Drawing for the job (mm, zero at the part's lowest x, y, z). A direction names the side the tool comes from. Round coordinates to 2 decimals unless told otherwise and drop trailing zeros. Loops run counter-clockwise (first coordinate to the right, second up) from the corner with the lowest first, then second, coordinate; pieces in that order, holes last. Notation, with made-up numbers: M -21.5,36 L 11.5,36 A15 ccw 11.5,64 Z; hole C 31.5,69.25 d4. An arc over 180 degrees is marked long. Put each result on its own line as item: value. Start each with the question number.
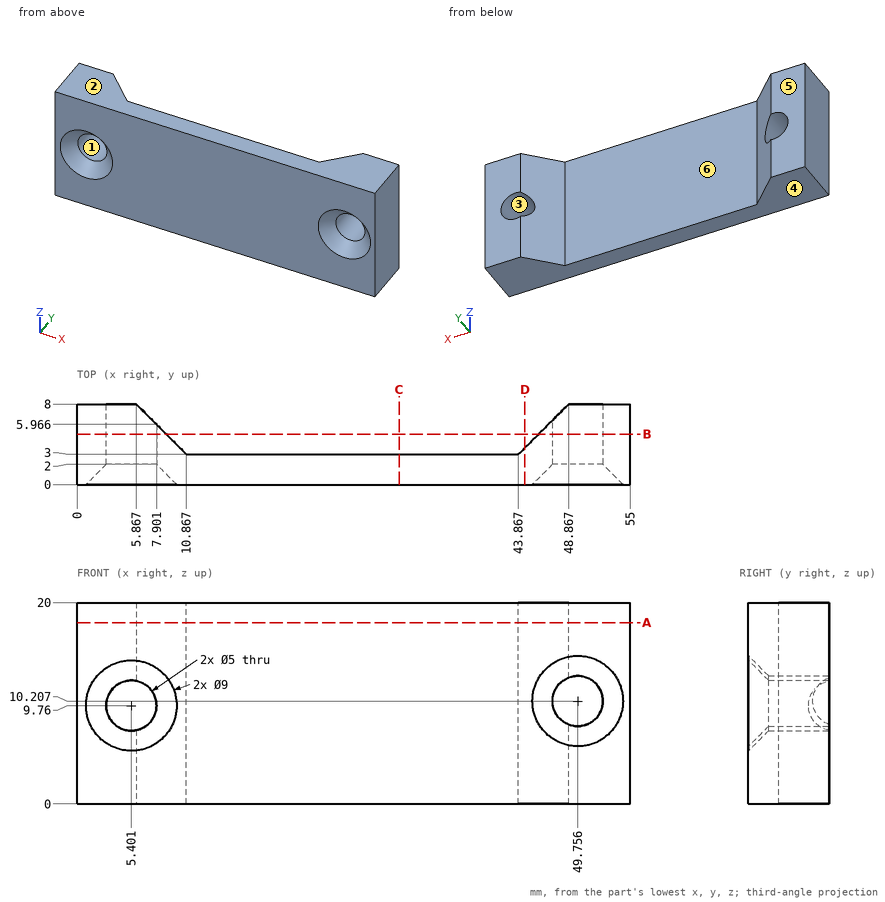
1. Cut at C-C, the plane x = 32. Give the cut face in (y, z).
2. Cut at B-B, the plane y = 5. Give the cut face in (x, z).
3. Which spindle directions (+Z, -Z, +X, -X, +Y, -Y) get a long thin tool onto all of the face, cutting with end or side? Do the marked faces 5 and 6. Say none if no direction does.
4. Mould opens along Z. For the marked faces 1, 2, 3 and 4 say: released by +Z, released by -Z, zero draft, split by the parting line, or undercut.
5. Cut at D-D, the plane x = 44.5. Give the cut face in (y, z).
6. Cut at A-A, the plane z = 18. Give the cut face in (x, y).
7. Wall check: L1, parallel to X at y = 3.25, z = 8.25 (1 decimal); L2, parallel to X at y = 3.75, z = 7.5 (1 decimal); L3, parallel to Y at x = 13.5, z = 12.25. Give the ranges that are in metal, low to high.
8. Drop flat-ended pins along their axis: pin 1 (4 mm diameter, centred on x = 5.4, z = 9.76, fed in from +Y); pin 2 (2 mm diameter, centred on x = 24.5, z = 16.5, fed in from +Y). Give the stop position or say it passes through.
Results list:
1. outline: M 0,0 L 3,0 L 3,20 L 0,20 Z
2. outline: M 0,0 L 8.87,0 L 8.87,20 L 0,20 Z; M 45.87,0 L 55,0 L 55,20 L 45.87,20 Z; hole C 5.4,9.76 d5; hole C 49.76,10.21 d5
3. face 5: +Z, -Z, +X, -X, +Y
3. face 6: +Z, -Z, +Y
4. face 1: undercut
4. face 2: released by +Z
4. face 3: undercut
4. face 4: released by -Z
5. outline: M 0,0 L 3.63,0 L 3.63,20 L 0,20 Z
6. outline: M 0,0 L 55,0 L 55,8 L 48.87,8 L 43.87,3 L 10.87,3 L 5.87,8 L 0,8 Z
7. L1: x = 0 to 3.4, 7.4 to 10.6, 44.1 to 48.2, 51.3 to 55
7. L2: x = 0 to 4.3, 6.5 to 10.1, 44.6 to 55
7. L3: y = 0 to 3
8. pin 1: passes through
8. pin 2: stops at y = 3
